from build123d import *

# Parameters (mm, degrees)
PAD_DEPTH         = 100
SKETCH001_W       = 13
SKETCH001_H       = 92
POCKET_DEPTH      = 13
SKETCH002_R       = 3.9
PAD001_DEPTH      = 15
PAD001_DEPTH_BACK = 115
FILLET_R          = 1
SKETCH003_R       = 2.5
PAD002_DEPTH      = 3
SKETCH004_R       = 1.25
POCKET001_DEPTH   = 10
POCKET002_DEPTH   = 130.001
POCKET003_DEPTH   = 0.801
POCKET004_DEPTH   = 0.801
POCKET005_DEPTH   = 0.801
POCKET006_DEPTH   = 0.801
SKETCH006_W       = 5
SKETCH006_H       = 14.5
PAD003_DEPTH      = 53.3
POCKET007_DEPTH   = 6.401
PAD004_DEPTH      = 14.5
POCKET008_DEPTH   = 14.5
FILLET001_R       = 5
FILLET002_R       = 5
FILLET003_R       = 10
FILLET004_R       = 5


with BuildPart() as part:
    # Sketch → Pad (new body)
    with BuildSketch(Plane.XY):
        Polygon((0, 0), (18, 0), (18, 5), (5, 18), (0, 18), align=None)
    extrude(amount=PAD_DEPTH)

    # Sketch001 (on Face4 of Pad) → Pocket (cut)
    with BuildSketch(Plane(origin=(0, 18, 0), x_dir=(-1, 0, 0), z_dir=(0, 1, 0))):
        with Locations((-11.5, 50)):
            Rectangle(SKETCH001_W, SKETCH001_H)
    extrude(amount=-POCKET_DEPTH, mode=Mode.SUBTRACT)

    # Sketch002 (on Face5 of Pocket) → Pad001 (join, two sides)
    with BuildSketch(Plane.XY.offset(100)) as pad001_sk:
        with Locations((3.9, 3.9)):
            Circle(SKETCH002_R)
    extrude(amount=PAD001_DEPTH)
    extrude(pad001_sk.sketch, amount=-PAD001_DEPTH_BACK)

    # Fillet
    fillet_edges = [part.edges().sort_by_distance(p)[0] for p in [
        (0, 3.9, 115),
        (0, 3.9, -15),
    ]]
    fillet(fillet_edges, radius=FILLET_R)

    # Sketch003 (on Face10 of Fillet) → Pad002 (join)
    with BuildSketch(Plane.XZ):
        with Locations((2.5, 93)):
            Circle(SKETCH003_R)
        with Locations((15, 93)):
            Circle(SKETCH003_R)
        with Locations((15, 72)):
            Circle(SKETCH003_R)
        with Locations((2.5, 72)):
            Circle(SKETCH003_R)
        with Locations((15, 7)):
            Circle(SKETCH003_R)
        with Locations((15, 28)):
            Circle(SKETCH003_R)
        with Locations((2.5, 7)):
            Circle(SKETCH003_R)
        with Locations((2.5, 28)):
            Circle(SKETCH003_R)
    extrude(amount=PAD002_DEPTH)

    # Sketch004 (on Face37 of Pad002) → Pocket001 (cut)
    with BuildSketch(Plane.XZ.offset(3)):
        with Locations((2.5, 93)):
            Circle(SKETCH004_R)
        with Locations((15, 93)):
            Circle(SKETCH004_R)
        with Locations((2.5, 72)):
            Circle(SKETCH004_R)
        with Locations((15, 72)):
            Circle(SKETCH004_R)
        with Locations((15, 28)):
            Circle(SKETCH004_R)
        with Locations((2.5, 28)):
            Circle(SKETCH004_R)
        with Locations((15, 7)):
            Circle(SKETCH004_R)
        with Locations((2.5, 7)):
            Circle(SKETCH004_R)
    extrude(amount=-POCKET001_DEPTH, mode=Mode.SUBTRACT)

    # Sketch005 (on Face51 of Pocket001) → Pocket002 (cut, through all)
    with BuildSketch(Plane.XY.offset(115)):
        with BuildLine():
            Line((4.680603, 7.721081), (18, 5))
            Line((18, 5), (18, 20))
            Line((-5, 20), (18, 20))
            Line((-5, 3.9), (-5, 20))
            Line((0, 3.9), (-5, 3.9))
            ThreePointArc((4.680603, 7.721081), (1.433662, 6.921122), (0, 3.9))
        make_face()
    extrude(amount=-POCKET002_DEPTH, mode=Mode.SUBTRACT)

    # Pocket002 Face15 → Pocket003 (cut, through all)
    with BuildSketch(Plane(origin=(2.572191, 7, 93), x_dir=(-1, 0, 0), z_dir=(0, -1, 0))):
        with BuildLine():
            ThreePointArc((1.038623, 0.792786), (-0.348796, 1.176975), (-1.177809, 0))
            ThreePointArc((-1.177809, 0), (-0.348796, -1.176975), (1.038623, -0.792786))
            Line((1.038623, -0.792786), (1.038623, 0.792786))
        make_face()
    extrude(amount=-POCKET003_DEPTH, mode=Mode.SUBTRACT)

    # Pocket003 Face15 → Pocket004 (cut, through all)
    with BuildSketch(Plane(origin=(2.572191, 7, 72), x_dir=(-1, 0, 0), z_dir=(0, -1, 0))):
        with BuildLine():
            ThreePointArc((1.038623, 0.792786), (-0.348796, 1.176975), (-1.177809, 0))
            ThreePointArc((-1.177809, 0), (-0.348796, -1.176975), (1.038623, -0.792786))
            Line((1.038623, -0.792786), (1.038623, 0.792786))
        make_face()
    extrude(amount=-POCKET004_DEPTH, mode=Mode.SUBTRACT)

    # Pocket004 Face21 → Pocket005 (cut, through all)
    with BuildSketch(Plane(origin=(2.572191, 7, 7), x_dir=(-1, 0, 0), z_dir=(0, -1, 0))):
        with BuildLine():
            ThreePointArc((1.038623, 0.792786), (-0.348796, 1.176975), (-1.177809, 0))
            ThreePointArc((-1.177809, 0), (-0.348796, -1.176975), (1.038623, -0.792786))
            Line((1.038623, -0.792786), (1.038623, 0.792786))
        make_face()
    extrude(amount=-POCKET005_DEPTH, mode=Mode.SUBTRACT)

    # Pocket005 Face24 → Pocket006 (cut, through all)
    with BuildSketch(Plane(origin=(2.572191, 7, 28), x_dir=(-1, 0, 0), z_dir=(0, -1, 0))):
        with BuildLine():
            ThreePointArc((1.038623, 0.792786), (-0.348796, 1.176975), (-1.177809, 0))
            ThreePointArc((-1.177809, 0), (-0.348796, -1.176975), (1.038623, -0.792786))
            Line((1.038623, -0.792786), (1.038623, 0.792786))
        make_face()
    extrude(amount=-POCKET006_DEPTH, mode=Mode.SUBTRACT)

    # Sketch006 (on Face30 of Pocket006) → Pad003 (join)
    with BuildSketch(Plane(origin=(0, 5, 0), x_dir=(-1, 0, 0), z_dir=(0, 1, 0))):
        with Locations((-3.9, -4.25)):
            Rectangle(SKETCH006_W, SKETCH006_H)
    extrude(amount=PAD003_DEPTH)

    # Sketch007 (on Face11 of Pad003) → Pocket007 (cut, through all)
    with BuildSketch(Plane.YZ.offset(6.4)):
        with BuildLine():
            Line((48.550002, -3.05), (50.050002, -3.05))
            ThreePointArc((50.050002, -8.95), (52.999998, -6), (50.050002, -3.05))
            Line((48.55, -8.95), (50.050002, -8.95))
            ThreePointArc((48.550002, -3.05), (45.600002, -5.999999), (48.55, -8.95))
        make_face()
    extrude(amount=-POCKET007_DEPTH, mode=Mode.SUBTRACT)

    # Pocket007 Face11 → Pad004 (add)
    with BuildSketch(Plane(origin=(6.4, 31.794028, -4.172133), x_dir=(0, -1, 0), z_dir=(1, 0, 0))):
        Polygon((24.424211, -7.172133), (24.424211, -4.172133), (24.900702, -4.172133), (24.900702, 7.327867), (-26.505972, 7.327867), (-26.505972, -7.172133), align=None)
        with BuildLine():
            Line((-16.755973, -1.122133), (-18.255973, -1.122133))
            ThreePointArc((-18.255973, -1.122133), (-21.205969, 1.827867), (-18.255973, 4.777867))
            Line((-18.255973, 4.777867), (-16.755972, 4.777867))
            ThreePointArc((-16.755972, 4.777867), (-13.805974, 1.827866), (-16.755973, -1.122133))
        make_face(mode=Mode.SUBTRACT)
    extrude(amount=PAD004_DEPTH)

    # Sketch008 (on Face18 of Pad004) → Pocket008 (cut)
    with BuildSketch(Plane(origin=(0, 0, -11.5), x_dir=(1, 0, 0), z_dir=(0, 0, -1))):
        Polygon((15.9, -58.3), (15.9, -38.3), (1.4, -13.185263), (-8.6, -13.185263), (-8.6, -68.3), (32.38311, -68.3), (32.38311, -6.893326), (6.4, -6.893326), (22.38311, -40.3), (22.38311, -58.3), align=None)
    extrude(amount=-POCKET008_DEPTH, mode=Mode.SUBTRACT)

    # Fillet001
    fillet001_edges = [part.edges().sort_by_distance(p)[0] for p in [
        (1.4, 13.185263, -4.25),
    ]]
    fillet(fillet001_edges, radius=FILLET001_R)

    # Fillet002
    fillet002_edges = [part.edges().sort_by_distance(p)[0] for p in [
        (15.9, 38.3, -4.25),
    ]]
    fillet(fillet002_edges, radius=FILLET002_R)

    # Fillet003
    fillet003_edges = [part.edges().sort_by_distance(p)[0] for p in [
        (20.9, 37.200117, -4.25),
    ]]
    fillet(fillet003_edges, radius=FILLET003_R)

    # Fillet004
    fillet004_edges = [part.edges().sort_by_distance(p)[0] for p in [
        (18.4, 58.3, -11.5),
        (18.4, 58.3, 3),
    ]]
    fillet(fillet004_edges, radius=FILLET004_R)


solid = part.part
Source: CAD feature listing. Evaluate the final solid. Frame: model axes, mm. A direction names the side the tool comes from. Give positions to 0.01 mm unless a question says otherwise; leave off trailing zeros. Write each loop counter-clockwise with the first axis right and the second up, starting at its lowest first coordinate (ties: lowest second). Pieces come first, ordered by that corner, then holes. Notation, with made-up numbers: M 69.25,-3.5 L 74.25,-3.5 A14 ccw 74.25,16.5 Z; hole C 14,60 d4. An arc over 180 degrees is marked long. Return JSON: item names as keys, results as strings. Group by question number.
1) Set-up query: faces 4 (the face through (18.4, 45.6, -6.1)), 5 (the face through (15.9, 49.1, -2.7)), 6 (the face through (6.677, 6.638, 50.644)), 7 (the face through (1, -3, 6)), 8 (the face through (14.46, -1.48, 69.56)). Return all of +Z, -Z, +X, -X, +Y, -Y with unobstructed straight access to the full face (end or side cutting, diameter ignored); none if empty.
2) Cut plane D-D, the plane y = 28.5. Output: boundary loops of the cut face in (x, z).
3) Ray query, L1, parallel to Z at x = 2.5, y = 4.25; L2, parallel to X at y = 3, z = 72; L3, parallel to Z at x = 15, y = 0.25. Return the intervals inside material, ascending.
4) First-contact query: pin 1 Ø2 at (x, y) = (14, 6) entering from -Z; pin 2 Ø1.7 at (x, y) = (18, 49) entering from +Z; pin 3 Ø3 at (x, z) = (15, 28) entering from +Y; pin 4 Ø2 at (x, y) = (10, 34) entering from -Z. Flat tips, straight axial feed; report the tip coordinate or a pass-through.
5) Cut plane C-C, the plane z = 103. Output: boundary loops of the cut face in (x, y).
6) Cut plane B-B, the plane y = 41. Output: boundary loops of the cut face in (x, z).
7) Draft query along Z for faces 1 (the face through (12.5, -1.5, 7.1)), 2 (the face through (1, -3, 27)), 3 (the face through (4, 4, 115)). Return one class per face: released by +Z, released by -Z, zero draft, split by the parting line, or undercut.
Data:
{
 "1": {"face 4": "+X, -X", "face 5": "+Z, -Z, -X, +Y", "face 6": "+X, +Y", "face 7": "+Z, -Z, +X, -X, -Y", "face 8": "-Y"},
 "2": {"outline": "M 10.24,-11.5 L 16.74,-11.5 L 16.74,3 L 10.24,3 Z"},
 "3": {"L1": "z = -15 to 5.75, 8.25 to 26.75, 29.25 to 70.75, 73.25 to 91.75, 94.25 to 115", "L2": "x = 0 to 1.25, 3.75 to 13.75, 16.25 to 18", "L3": "z = 0 to 5.75, 8.25 to 26.75, 29.25 to 70.75, 73.25 to 91.75, 94.25 to 100"},
 "4": {"pin 1": "stops at z = 0", "pin 2": "stops at z = 3", "pin 3": "stops at y = 5", "pin 4": "passes through"},
 "5": {"outline": "C 3.9,3.9 d7.8"},
 "6": {"outline": "M 15.9,-11.5 L 20.9,-11.5 L 20.9,3 L 15.9,3 Z"},
 "7": {"face 1": "undercut", "face 2": "zero draft", "face 3": "released by +Z"}
}
